CAD build for the part. Positions are in the model's coordinates, mm. Round coordinates to 2 decimals unless told otherwise and drop trailing zeros. Loops run counter-clockwise (first coordinate to the right, second up) from the corner with the lowest first, then second, coordinate; pieces in that order, holes last. Notation, with made-up numbers: M 81.5,35 L 112.5,35 A5 ccw 112.5,40 Z; hole C 23.5,13 d7. An arc over 180 degrees is marked long. Use one line per item in the form item = value.
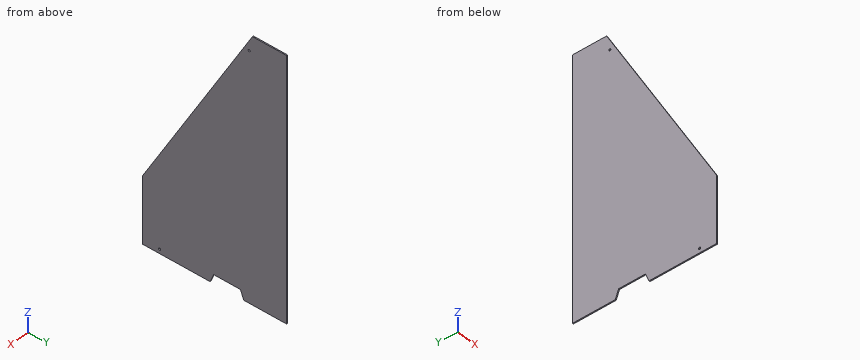
Autodesk Inventor part; units mm, degrees
ref_plane "YZ Plane" through (0, 0, 0) normal (1, 0, 0) x (0, 1, 0)
ref_plane "XZ Plane" through (0, 0, 0) normal (0, 1, 0) x (-1, 0, 0)
ref_plane "XY Plane" through (0, 0, 0) normal (0, 0, 1) x (1, 0, 0)
sketch "Sketch1" plane through (0, 0, 0) normal (1, 0, 0) x (0, 1, 0)
  line L0 (0, 0) -> (-127, 0)
  line L1 (0, 0) -> (127, 0) construction
  line L2 (-227.417, 0) -> (-428.6358, 0)
  line L3 (0, 0) -> (0, 762)
  line L4 (0, 0) -> (762, 0) construction
  line L5 (0, 762) -> (-101.6, 762)
  line L6 (-101.6, 762) -> (-428.6358, 193.675)
  line L7 (-428.6358, 193.675) -> (-428.6358, 0)
  line L8 (-127, 0) -> (-137.521, 25.4)
  line L9 (-127, 0) -> (-99.5072, 0) construction
  line L10 (-137.521, 25.4) -> (-216.896, 25.4)
  line L11 (-216.896, 25.4) -> (-227.417, 0)
  dimension "d0" = 127
  dimension "d1" = 180
  dimension "d8" = 201.2188
  dimension "d10" = 762
  dimension "d11" = 90
  dimension "d13" = 90
  dimension "d14" = 90
  dimension "d18" = 112.5
  dimension "d19" = 79.375
  dimension "d20" = 112.5
  dimension "d21" = 112.5
  dimension "d22" = 25.4
  dimension "d23" = 0
  dimension "d35" = 101.6
  dimension "d36" = 193.675
extrude "Extrusion1" add sketch "Sketch1" along normal blind 3.175
sketch "Sketch2" plane through (0, 0, 0) normal (-1, 0, 0) x (0, 0, 1)
  line L0 (0, 0) -> (0, -127)
  line L1 (0, -127) -> (25.4, -137.521)
  line L2 (25.4, -137.521) -> (25.4, -216.896)
  line L3 (25.4, -216.896) -> (0, -227.417)
  line L4 (0, -227.417) -> (0, -428.6358)
  line L5 (0, -428.6358) -> (193.675, -428.6358)
  line L6 (193.675, -428.6358) -> (762, -101.6)
  line L7 (762, -101.6) -> (762, 0)
  line L8 (762, 0) -> (0, 0)
  point P0 (12.7, -377.8358)
  point P1 (717.55, -111.125)
  dimension "d24" = 111.125
  dimension "d25" = 44.45
  dimension "d26" = 50.8
  dimension "d27" = 12.7
hole "Hole1" at (0, -377.8358, 12.7) at (0, -111.125, 717.55) direction (1, 0, 0) diameter 6.35 end through all
properties part number "side panel" material "Polycarbonate, Clear"
1. Cut at A-A on x = 1.25. Write the cut outline in (y, z) (3 decimals), and give its area (3 significant figures).
Completed:
outline = M -428.636,0 L -227.417,0 L -216.896,25.4 L -137.521,25.4 L -127,0 L 0,0 L 0,762 L -101.6,762 L -428.636,193.675 Z; hole C -377.836,12.7 d6.35; hole C -111.125,717.55 d6.35
area = 231,000 mm2
2. Cut at C-C on y = -294. Write the cut outline in (x, z) (3 decimals).
Completed:
outline = M 0,0 L 3.175,0 L 3.175,427.646 L 0,427.646 Z
3. Probe line 1 along Y through (x, z) = (2.55, 12.7); line 2 along Y through (x, z) = (1.8, 716); line 3 along Y through (x, z) = (2, 717.55). List the from-to ranges inside material, lowest first. Write a range as from..to.
Completed:
line_1 = -428.64..-381.01, -374.66..-222.16, -132.26..0
line_2 = -128.07..-113.9, -108.35..0
line_3 = -127.18..-114.3, -107.95..0
4. Cut at B-B on z = 421. Write the cut outline in (x, y) (3 decimals), and give its area (3 significant figures).
Completed:
outline = M 0,-297.824 L 3.175,-297.824 L 3.175,0 L 0,0 Z
area = 946 mm2
5. Drop a flat-ended pin along its axis: P1, Ø1, axis at x = 2, y = -161, coming from the -Z side. Give the stop position or say it passes through.
Completed:
P1 = 25.4
